Study the drawing (mm; zero at the part's minimum x, y, z) and answer. Give positions to 0.01 mm unless a question says otherwise; leave off trailing zeros. Order: outer loops, then holes, each group sorted by start corner. A loop starts at its lowest first (then second) coordinate and runs counter-clockwise, first axis right, second up.
Item 1: A cutting plane is placed at C-C (z = 960). Write down the section's boundary in (x, y) (3 decimals), plus the area to 3 significant figures.
Item 2: Find the intervals of material crossed by line 1 along Z through (x, y) = (277.5, 3.25); line 2 along Z through (x, y) = (461.5, 9.75); line 3 along X through (y, z) = (10.25, 1104), in increasing order.
Item 3: Given pin 1 Ø5 at (x, y) = (484, 9) entering from +Z; pin 2 Ø8 at (y, z) = (10.5, 1082) entering from -X, each flat-ended and moving along its own axis, determine where each tip first touches the part or whether it passes through.
Item 4: A cutting plane is placed at B-B (z = 1147). Write down the section's boundary in (x, y) (3 decimals), plus the area to 3 significant figures.
Item 5: A cutting plane is placed at A-A (y = 7). Write down the section's boundary in (x, z).
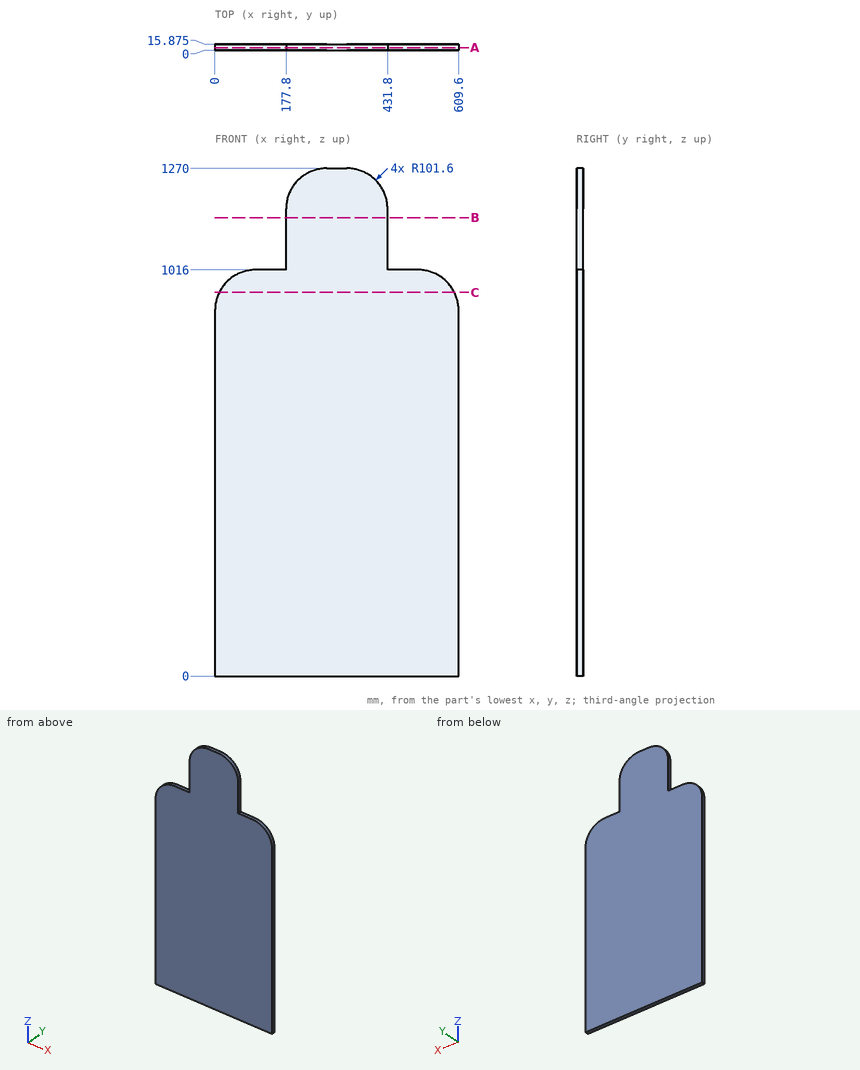
Response values:
1. outline: (10.808, 0) - (598.792, 0) - (598.792, 15.875) - (10.808, 15.875) - close
1. area: 9,330 mm2
2. line 1: z = 0 to 1269.98
2. line 2: z = 0 to 1016
2. line 3: x = 177.8 to 431.8
3. pin 1: stops at z = 1016
3. pin 2: stops at x = 177.8
4. outline: (177.8, 0) - (431.8, 0) - (431.8, 15.875) - (177.8, 15.875) - close
4. area: 4,030 mm2
5. outline: (0, 0) - (609.6, 0) - (609.6, 914.4) arc R101.6 ccw to (508, 1016) - (431.8, 1016) - (431.8, 1168.4) arc R101.6 ccw to (330.2, 1270) - (279.4, 1270) arc R101.6 ccw to (177.8, 1168.4) - (177.8, 1016) - (101.6, 1016) arc R101.6 ccw to (0, 914.4) - close
